Geometry check sheet. Reference: the model listing, model coordinates, mm. A direction names the side the tool comes from. Coordinates: 2 decimals unless noted, no trailing zeros. Loops run counter-clockwise (first coordinate to the right, second up) from the corner with the lowest first, then second, coordinate; pieces in that order, holes last. Notation, with made-up numbers: (56, 65.25) - (88, 65.25) arc R12 cw to (88, 76.25) - close; hole circle Ø1 at (-17.75, 79.25). An arc over 180 degrees is marked (long way). One line per item, written item: value.
from build123d import *
from build123d.topology import SkipClean

# Parameters (mm, degrees)
SKETCH1_R               = 44.5
SKETCH1_R_2             = 38.5
BOSS_EXTRUDE1_DEPTH     = 8
SKETCH2_R               = 2
BOSS_EXTRUDE2_DEPTH     = 8
CIRPATTERN3_COUNT       = 4
BOSS_EXTRUDE3_START     = -50
SKETCH5_R               = 44.5
SKETCH5_R_2             = 38.5
BOSS_EXTRUDE3_DEPTH     = 50
BOSS_EXTRUDE4_START     = -50
BOSS_EXTRUDE4_OUTLINE_R = 2
BOSS_EXTRUDE4_DEPTH     = 50
CIRPATTERN4_COUNT       = 4
CUT_EXTRUDE2_START      = 41
CUT_EXTRUDE2_DEPTH      = 41
CIRPATTERN5_COUNT       = 4
SKETCH9_R               = 5.5
CUT_EXTRUDE3_DEPTH      = 4
CIRPATTERN6_COUNT       = 4


# Read off the part's stored shape, not the designer's step: Boss-Extrude4
with BuildPart() as part:
    # Sketch1 → Boss-Extrude1 (new body)
    with BuildSketch(Plane(origin=(0, 0, 0), x_dir=(1, 0, 0), z_dir=(0, 1, 0))):
        with Locations(Location((0, 0, 0), (0, 0, 270))):
            Circle(SKETCH1_R)
        with Locations(Location((0, 0, 0), (0, 0, 270))):
            Circle(SKETCH1_R_2, mode=Mode.SUBTRACT)
    extrude(amount=BOSS_EXTRUDE1_DEPTH)

    # Sketch2 → Boss-Extrude2 (add)
    with BuildSketch(Plane(origin=(0, 0, 0), x_dir=(1, 0, 0), z_dir=(0, 1, 0))):
        with BuildLine():
            Line((41.951101238, 14.844362731), (101.951101238, 14.844362731))
            Line((101.951101238, 14.844362731), (101.951101238, -14.844362731))
            Line((101.951101238, -14.844362731), (41.951101238, -14.844362731))
            ThreePointArc((41.951101238, -14.844362731), (44.5, 0), (41.951101238, 14.844362731))
        make_face()
        with Locations(Location((90.951101238, 0, 0), (0, 0, 270))):
            Circle(SKETCH2_R, mode=Mode.SUBTRACT)
    boss_extrude2 = extrude(amount=BOSS_EXTRUDE2_DEPTH)

    # CirPattern3: Boss-Extrude2 ×4 about axis
    cirpattern3_axis = Axis((0, 0, 0), (0, 1, 0))
    for i in range(1, CIRPATTERN3_COUNT):
        add(boss_extrude2.rotate(cirpattern3_axis, i * 360 / CIRPATTERN3_COUNT))

    # Sketch5 → Boss-Extrude3 (add)
    with SkipClean():  # the faces are left unmerged after this step: merging them gives an invalid solid
        with BuildSketch(Plane(origin=(0, 0, 0), x_dir=(1, 0, 0), z_dir=(0, 1, 0)).offset(BOSS_EXTRUDE3_START)):
            with Locations(Location((0, 0, 0), (0, 0, 70.513716386))):
                Circle(SKETCH5_R)
            with Locations(Location((0, 0, 0), (0, 0, 270))):
                Circle(SKETCH5_R_2, mode=Mode.SUBTRACT)
        extrude(amount=BOSS_EXTRUDE3_DEPTH)
    add(part.part.scale(1), mode=Mode.REPLACE)  # the faces are merged on a copy

    # Boss-Extrude4 outline → Boss-Extrude4 (add)
    with BuildSketch(Plane(origin=(0, 0, 0), x_dir=(1, 0, 0), z_dir=(0, 1, 0)).offset(BOSS_EXTRUDE4_START)):
        with BuildLine():
            Line((41.951101238, -14.844362731), (57.951101238, -14.844362731))
            ThreePointArc((57.951101238, -14.844362731), (61.83977211, 0), (57.951101238, 14.844362731))
            Line((57.951101238, 14.844362731), (41.951101238, 14.844362731))
            ThreePointArc((41.951101238, 14.844362731), (44.5, 0), (41.951101238, -14.844362731))
        make_face()
        with Locations((51.9, 0)):
            Circle(BOSS_EXTRUDE4_OUTLINE_R, mode=Mode.SUBTRACT)
    boss_extrude4 = extrude(amount=BOSS_EXTRUDE4_DEPTH)

    # CirPattern4: Boss-Extrude4 ×4 about axis
    cirpattern4_axis = Axis((0, 0, 0), (0, 1, 0))
    for i in range(1, CIRPATTERN4_COUNT):
        add(boss_extrude4.rotate(cirpattern4_axis, i * 360 / CIRPATTERN4_COUNT))

    # Sketch8 → Cut-Extrude2 (cut)
    with BuildSketch(Plane.XZ.offset(CUT_EXTRUDE2_START)):
        with BuildLine():
            Line((61.239313057, -6), (45.9, -6))
            Line((45.9, -6), (45.9, 6))
            Line((45.9, 6), (61.239313057, 6))
            ThreePointArc((61.239313057, 6), (61.83977211, 0), (61.239313057, -6))
        make_face()
    cut_extrude2 = extrude(amount=-CUT_EXTRUDE2_DEPTH, mode=Mode.SUBTRACT)

    # CirPattern5: Cut-Extrude2 ×4 about axis
    cirpattern5_axis = Axis((0, 0, 0), (0, 1, 0))
    for i in range(1, CIRPATTERN5_COUNT):
        add(cut_extrude2.rotate(cirpattern5_axis, i * 360 / CIRPATTERN5_COUNT), mode=Mode.SUBTRACT)

    # Sketch9 → Cut-Extrude3 (cut)
    with BuildSketch(Plane(origin=(0, 8, 0), x_dir=(1, 0, 0), z_dir=(0, 1, 0))):
        with Locations(Location((90.951101238, 0, 0), (0, 0, 270))):
            Circle(SKETCH9_R)
    cut_extrude3 = extrude(amount=-CUT_EXTRUDE3_DEPTH, mode=Mode.SUBTRACT)

    # CirPattern6: Cut-Extrude3 ×4 about axis
    cirpattern6_axis = Axis((0, 0, 0), (0, 1, 0))
    for i in range(1, CIRPATTERN6_COUNT):
        add(cut_extrude3.rotate(cirpattern6_axis, i * 360 / CIRPATTERN6_COUNT), mode=Mode.SUBTRACT)


solid = part.part
(1) Material ranges on probe 1 along X at (y, z) = (-44, 0); probe 2 along Y at (x, z) = (-57, -3); probe 3 along X at (y, z) = (-20, 0), recorded low to high. Write a range as from..to.
Reply:
probe 1: -61.84..-53.9, -49.9..-38.5, 38.5..49.9, 53.9..61.84
probe 2: -50..-41, 0..8
probe 3: -45.9..-38.5, 38.5..45.9
(2) Cross-section at D-D on x = -75. Record the cut outline in (y, z), and give its area (3 significant figures).
Reply:
outline: (0, -14.84) - (8, -14.84) - (8, 14.84) - (0, 14.84) - close
area: 238 mm2
(3) Cross-section at C-C on z = 83. Record the cut outline in (x, y).
Reply:
outline: (-14.84, 0) - (14.84, 0) - (14.84, 8) - (-14.84, 8) - close
(4) Go/stop test with flat-tipped pins: pin 1 Ø3.5 at (x, z) = (0.5, 90.5) entering from +Y; pin 2 Ø6 at (x, z) = (79, 1.5) entering from -Y; pin 3 Ø13 at (y, z) = (-18, 2) entering from +X. Record where each tip stops, or that it passes through.
Reply:
pin 1: y = 4
pin 2: y = 0
pin 3: x = 61.24
(5) Release check for a two-part mould opening along X. For faces 4 (the face through (0, 0, 80)), 5 (the face through (-54, -21, 6)), 6 (the face through (-45.9, -21, 0)) record: pulls with the +X half, pulls with the -X half, needs draft (parallel to the pull), parting line crosses it, or undercut.
Reply:
face 4: undercut
face 5: needs draft
face 6: pulls with the -X half
(6) Cross-section at B-B on x = 19. Record the cut outline in (y, z), and give its area (3 significant figures).
Reply:
outline: (-50, -40.24) - (8, -40.24) - (8, -33.49) - (-50, -33.49) - close; (-50, 33.49) - (8, 33.49) - (8, 40.24) - (-50, 40.24) - close
area: 784 mm2
(7) Access from +Z, -Z, +X, -X, +Y, -Y to the whole of each face (thin tool, end or side, straight path). Record for faces 1 (the face through (-0.1, 4, -88.6)), 2 (the face through (-56, -13, -14.844)), 3 (the face through (-6, -21, -54)).
Reply:
face 1: +Y
face 2: -Z, -X, +Y, -Y
face 3: -Z
